Read the model definition and answer for the solid it produces. Units are mm, in the model's axes. Face numbers are marked on the shaded views. Round coordinates to 2 decimals unless told otherwise and drop trailing zeros. Order: outer loops, then holes, each group sorted by start corner. A loop starts at its lowest first (then second) coordinate and runs counter-clockwise, first axis right, second up. Notation, with made-up numbers: (-29, 2) -> (-9, 2) arc R32 cw to (-9, 34) -> close; hole circle Ø9 at (34, 54). An arc over 180 degrees is marked (long way). Answer as a JSON object with one key per item and string values. Group by question number.
Item 1: Given P1, Ø2, axis at x = 23.5, z = 44, coming from the -Y side; P2, Ø4, axis at y = -2, z = 49.5, coming from the +X side; P3, Ø3, axis at y = 6.5, z = 19, coming from the +X side, each flat-ended and moving along its own axis, determine where each tip first touches the part or whether it passes through.
Item 2: Section B-B, the plane z = -1.5 is taken. Write down the section's boundary in (x, y).
Item 3: The mould has two halves that part along X. Classify the marked faces 1, 2 and 3: pulls with the +X half, pulls with the -X half, needs draft (parallel to the pull), parting line crosses it, or undercut.
Item 4: Consider probe 1 along Z at (x, y) = (-6, -6.5); probe 2 along Y at (x, z) = (1, -4.5); probe 3 along Y at (x, z) = (-11.5, 11). Determine where each line is inside the solid, lowest interval first. Write a range as from..to.
Item 5: Section A-A, the plane z = 40.5 is taken. Write down the section's boundary in (x, y).
from build123d import *

# Parameters (mm, degrees)
F3_C1_SIZE2 = 0.25
F3_C1_SIZE  = 0.5
F3_C2_SIZE2 = 0.25
F3_C2_SIZE  = 0.5


# Not quite as in the source:
# - a fillet or chamfer that OpenCascade refuses, or shapes differently, is made with other operations: its cross-section is extruded or revolved along the edge and cut away or added


with BuildPart() as f1:
    # F0 (on Front) → F1 (revolve)
    with BuildSketch(Plane.XZ):
        Polygon((-24.2239079518, 85.7203521749), (-25.0227362253, 85.6770823112), (-23.5166698694, 57.8727796674), (-20.7616358603, 55.1226193476), (-17.0000027865, -14.3229160458), (2.9999972135, -14.3229160458), (2.9999972135, -13.5229167386), (-16.2421640236, -13.5229167386), (-19.9793957734, 55.4721326625), (-22.7344297825, 58.2222929823), align=None)
    revolve(axis=Axis((2.9999972135, 0, 16.662178661), (0, 0, -1)))

    # F2: fillet of radius 1 on 2 edges, made by hand

    # F2_s1 → F2_t2 (revolve, cut)
    with BuildSketch(Plane.XZ):
        with BuildLine():
            ThreePointArc((-24.2239458394, 85.7204973112), (-24.7789966166, 85.342605366), (-24.9698980485, 84.6988349638))
            Line((-24.9698980485, 84.6988349638), (-24.9898687726, 84.6977532163))
            ThreePointArc((-24.9898687726, 84.6977532163), (-25.0162129708, 85.1868809465), (-25.0427069494, 85.6760005637))
            Line((-25.0427069494, 85.6760005637), (-25.0238179728, 85.6970530353))
            ThreePointArc((-25.0238179728, 85.6970530353), (-24.6244188052, 85.7186871564), (-24.2289975194, 85.7398488106))
            Line((-24.2289975194, 85.7398488106), (-24.2239458394, 85.7204973112))
        make_face()
    revolve(axis=Axis((2.9999972135, 0, 85.6770823112), (0, 0, -1)), mode=Mode.SUBTRACT)

    # F2_s3 → F2_t4 (revolve, cut)
    with BuildSketch(Plane.XZ):
        with BuildLine():
            ThreePointArc((-17.0513818139, -13.3771534223), (-16.7405637995, -14.0490437922), (-16.0528456074, -14.3230660458))
            Line((-16.0528456074, -14.3230660458), (-16.0528456074, -14.3430660458))
            ThreePointArc((-16.0528456074, -14.3430660458), (-16.526424197, -14.3429160458), (-17.0000027865, -14.3429160458))
            Line((-17.0000027865, -14.3429160458), (-17.0199735106, -14.3239977933))
            ThreePointArc((-17.0199735106, -14.3239977933), (-17.0455881341, -13.851112425), (-17.071352538, -13.3782351698))
            Line((-17.071352538, -13.3782351698), (-17.0513818139, -13.3771534223))
        make_face()
    revolve(axis=Axis((2.9999972135, 0, -14.3229160458), (0, 0, -1)), mode=Mode.SUBTRACT)

    # F3: chamfer of 0.25 x 0.5 on 3 edges, made by hand

    # F3_c1
    f3_c1_edges = [f1.edges().sort_by_distance(p)[0] for p in [
        (26.7616302873, 0, 55.1226193476),
    ]]
    f3_c1_side = f1.faces().sort_by_distance((26.7651689498, 0, 55.1261517501))[0]
    chamfer(f3_c1_edges, length=F3_C1_SIZE, length2=F3_C1_SIZE2, reference=f3_c1_side)

    # F3_c2
    f3_c2_edges = [f1.edges().sort_by_distance(p)[0] for p in [
        (29.5166642964, 0, 57.8727796674),
    ]]
    f3_c2_side = f1.faces().sort_by_distance((29.5131256339, 0, 57.8692472648))[0]
    chamfer(f3_c2_edges, length=F3_C2_SIZE, length2=F3_C2_SIZE2, reference=f3_c2_side)


solid = f1.part
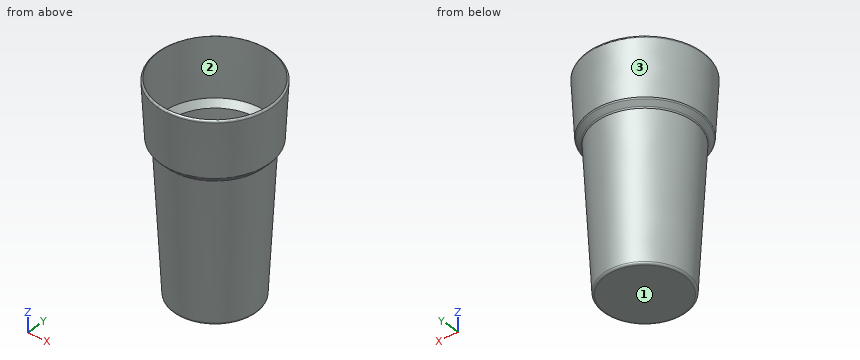
Values found:
{
 "1": {"P1": "y = -12.5", "P2": "x = 26.53", "P3": "x = 24.23"},
 "2": {"outline": "circle Ø41.39 at (3, 0); hole circle Ø39.79 at (3, 0)"},
 "3": {"face 1": "needs draft", "face 2": "undercut", "face 3": "parting line crosses it"},
 "4": {"probe 1": "-14.32..-13.52", "probe 2": "-20.43..-19.63, 19.63..20.43", "probe 3": "-15.7..-14.59, 14.59..15.7"},
 "5": {"outline": "circle Ø45.94 at (3, 0); hole circle Ø44.34 at (3, 0)"}
}
